```python
from build123d import *

# Parameters (mm, degrees)
SKETCH_1_W               = 120
SKETCH_1_H               = 80
EXTRUDE_1_DEPTH          = 50
SHELL_1_T                = -2.5
SKETCH_2_W               = 15
SKETCH_2_H               = 40
CUT_EXTRUDE_1_DEPTH      = 90
CUT_EXTRUDE_3_DEPTH      = 1
CUT_EXTRUDE_3_DEPTH_BACK = 81


with BuildPart() as part:
    # 草圖1 → 填料-伸長1 (new body)
    with BuildSketch(Plane.XY):
        Rectangle(SKETCH_1_W, SKETCH_1_H)
    extrude(amount=EXTRUDE_1_DEPTH)

    # 薄殼1
    shell_1_openings = [part.faces().sort_by_distance(p)[0] for p in [
        (0, 0, 50),
    ]]
    offset(amount=SHELL_1_T, openings=shell_1_openings, kind=Kind.INTERSECTION)

    # 草圖2 → 除料-伸長1 (cut)
    with BuildSketch(Plane.XZ.offset(40)):
        with Locations((-42.5, 30)):
            Rectangle(SKETCH_2_W, SKETCH_2_H)
    extrude(amount=-CUT_EXTRUDE_1_DEPTH, mode=Mode.SUBTRACT)

    # 草圖3 → 除料-伸長3 (cut, two sides)
    with BuildSketch(Plane.XZ.offset(40)) as cut_extrude_3_sk:
        with BuildLine():
            Line((43.6, 50), (43.6, 12.5))
            ThreePointArc((43.6, 12.5), (46.8, 9.3), (50, 12.5))
            Line((50, 12.5), (50, 50))
            Line((50, 50), (43.6, 50))
        make_face()
    extrude(amount=CUT_EXTRUDE_3_DEPTH, mode=Mode.SUBTRACT)
    extrude(cut_extrude_3_sk.sketch, amount=-CUT_EXTRUDE_3_DEPTH_BACK, mode=Mode.SUBTRACT)


solid = part.part
```
Verification items for the finished model (mm, model axes). A direction names the side the tool comes from. Coordinates: 2 decimals unless noted, no trailing zeros. Write each loop counter-clockwise with the first axis right and the second up, starting at its lowest first coordinate (ties: lowest second). Pieces come first, ordered by that corner, then holes. Notation, with made-up numbers: M 58.5,60 L 87.5,60 A20 cw 87.5,64 Z; hole C -13.75,12 d1. An arc over 180 degrees is marked long. One line per item, written item: value.
Item 1: Gauge pin test, flat ends, axial feed: pin 1 Ø5 at (x, y) = (13.5, -19) entering from +Z; pin 2 Ø0.8 at (x, y) = (-43.5, -39) entering from +Z. Record the tip position at first contact, or that the pin passes through.
Check sheet entries:
pin 1: stops at z = 2.5
pin 2: stops at z = 10
Item 2: Mould release check, pull along Y, two halves, no side actions. Record for faces 1 (the flat face through (-1, 37.5, 26)), 2 (the flat face through (-1, -40, 25)), 3 (the flat face through (60, -1, 25)): pulls with the +Y half, pulls with the -Y half, needs draft (parallel to the pull), parting line crosses it, or undercut.
Check sheet entries:
face 1: undercut
face 2: pulls with the -Y half
face 3: needs draft
Item 3: Scan lines: line 1 along Y through (x, z) = (32.5, 34); line 2 along X through (y, z) = (-4, 8.5); line 3 along Z through (x, y) = (-26, 24). Record each from-to range of solid material in increasing order.
Check sheet entries:
line 1: y = -40 to -37.5, 37.5 to 40
line 2: x = -60 to -57.5, 57.5 to 60
line 3: z = 0 to 2.5
Item 4: Access from +Z, -Z, +X, -X, +Y, -Y to the whole of each face (thin tool, end or side, straight path). Record for faces 4 (the flat face through (4, 39, 50)), 5 (the flat face through (-1, 1, 2.5)), 6 (the flat face through (-35, -39, 30)).
Check sheet entries:
face 4: +Z, +X, -X, +Y, -Y
face 5: +Z
face 6: +Z, +Y, -Y
Item 5: Section check C-C, the plane y = -34. Record the boundary of the cut face in (x, z), plus the area to 4 significant figures.
Check sheet entries:
outline: M -60,0 L 60,0 L 60,50 L 57.5,50 L 57.5,2.5 L -57.5,2.5 L -57.5,50 L -60,50 Z
area: 537.5 mm^2
Item 6: Section check B-B, the plane x = 46.8. Record the boundary of the cut face in (y, z).
Check sheet entries:
outline: M -40,0 L 40,0 L 40,9.3 L 37.5,9.3 L 37.5,2.5 L -37.5,2.5 L -37.5,9.3 L -40,9.3 Z
Item 7: Section check A-A, the plane z = 37. Record the boundary of the cut face in (x, y), plus the area to 3 significant figures.
Check sheet entries:
outline: M -60,-40 L -50,-40 L -50,-37.5 L -57.5,-37.5 L -57.5,37.5 L -50,37.5 L -50,40 L -60,40 Z; M -35,-40 L 43.6,-40 L 43.6,-37.5 L -35,-37.5 Z; M -35,37.5 L 43.6,37.5 L 43.6,40 L -35,40 Z; M 50,-40 L 60,-40 L 60,40 L 50,40 L 50,37.5 L 57.5,37.5 L 57.5,-37.5 L 50,-37.5 Z
area: 868 mm^2
